For this review, use the dimensioned drawing (mm, ordinates from the lowest corner) and the shaded views. Round coordinates to 2 decimals unless told otherwise and drop trailing zeros. Loops run counter-clockwise (first coordinate to the right, second up) from the corner with the lowest first, then second, coordinate; pieces in that order, holes last. Notation, with made-up numbers: M 85,48.5 L 96,48.5 A13 cw 96,60.5 Z; hole C -37.5,-25 d1. An arc over 180 degrees is marked long. Use a Markdown table: item, result. Add a question column.
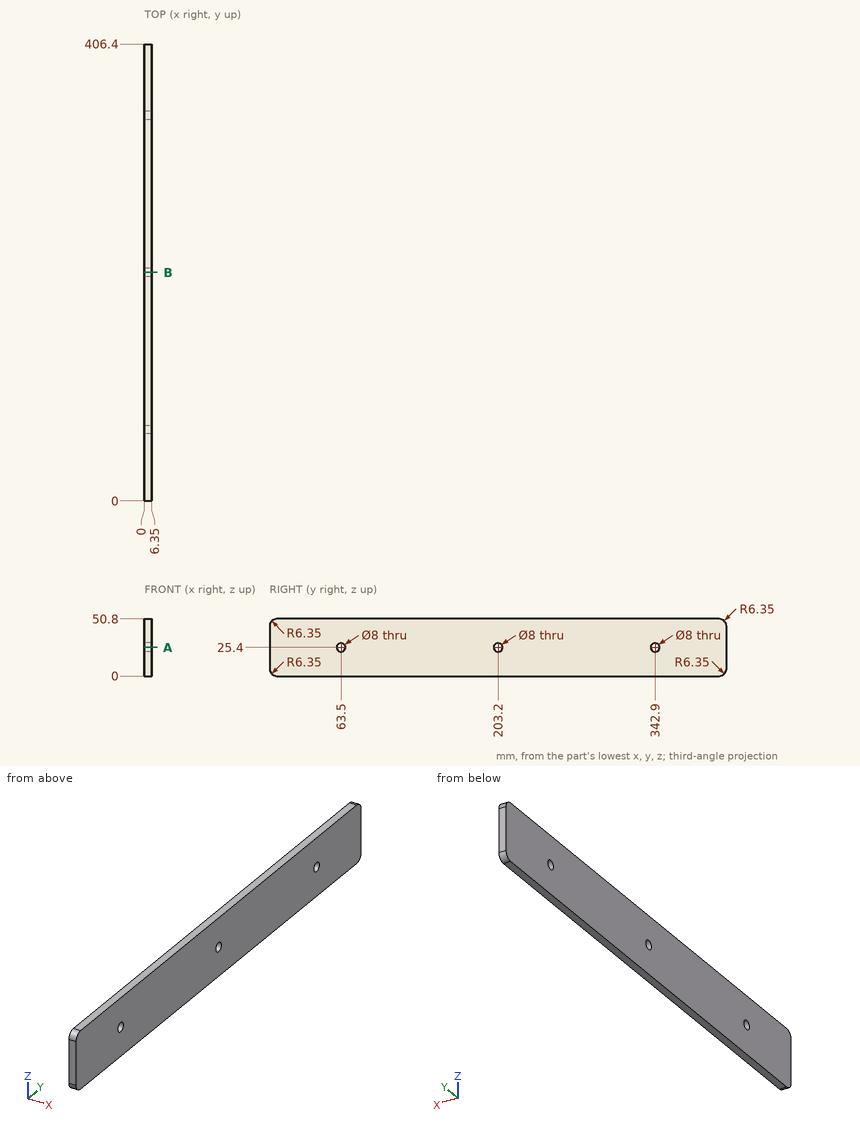
(1) Consider section B-B, the plane y = 203.2. Give the boundary of the cut face in (x, z), then the cut area to 3 significant figures.
(2) To check wall thickness, follow probe 1 along Z at (x, y) = (3.5, 342.9); probe 2 along Y at (x, z) = (4.75, 23.5); probe 3 along Y at (x, z) = (0.5, 24). State the ranges of each line that lie inside material, in increasing order.
(3) Insertion check: pin 1 Ø1.5 at (y, z) = (143.5, 33.5) entering from -X; pin 2 Ø6.5 at (y, z) = (342.9, 25.4) entering from +X. Each pin has a flat end and moves straight along its axis. Give the tip position at first contact, or say it passes through.
(4) Consider section A-A, the plane z = 25.4. Give the boundary of the cut face in (x, y), then the cut area to 3 significant figures.
Found:
| question | item | result |
|---|---|---|
| 1 | outline | M 0,0 L 6.35,0 L 6.35,21.4 L 0,21.4 Z; M 0,29.4 L 6.35,29.4 L 6.35,50.8 L 0,50.8 Z |
| 1 | area | 272 mm^2 |
| 2 | probe 1 | z = 0 to 21.4, 29.4 to 50.8 |
| 2 | probe 2 | y = 0 to 59.98, 67.02 to 199.68, 206.72 to 339.38, 346.42 to 406.4 |
| 2 | probe 3 | y = 0 to 59.75, 67.25 to 199.45, 206.95 to 339.15, 346.65 to 406.4 |
| 3 | pin 1 | stops at x = 0 |
| 3 | pin 2 | passes through |
| 4 | outline | M 0,0 L 6.35,0 L 6.35,59.5 L 0,59.5 Z; M 0,67.5 L 6.35,67.5 L 6.35,199.2 L 0,199.2 Z; M 0,207.2 L 6.35,207.2 L 6.35,338.9 L 0,338.9 Z; M 0,346.9 L 6.35,346.9 L 6.35,406.4 L 0,406.4 Z |
| 4 | area | 2,430 mm^2 |
